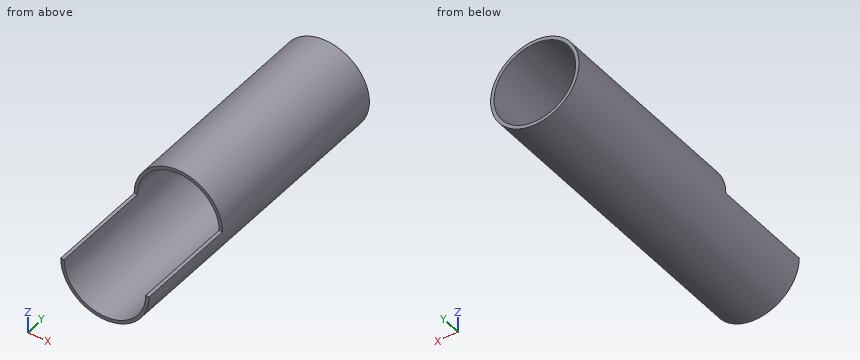
from build123d import *

# Parameters (mm, degrees)
SKETCH1_R           = 25.4
BOSS_EXTRUDE1_DEPTH = 180
SKETCH2_R           = 23.45
CUT_EXTRUDE1_DEPTH  = 180
SKETCH4_W           = 79.8
SKETCH4_H           = 60
CUT_EXTRUDE2_DEPTH  = 50


with BuildPart() as part:
    # Sketch1 → Boss-Extrude1 (new body)
    with BuildSketch(Plane(origin=(0, 0, 0), x_dir=(1, 0, 0), z_dir=(0, 1, 0))):
        with Locations(Location((0, 0, 0), (0, 0, 180))):
            Circle(SKETCH1_R)
    extrude(amount=BOSS_EXTRUDE1_DEPTH)

    # Sketch2 → Cut-Extrude1 (cut)
    with BuildSketch(Plane(origin=(0, 180, 0), x_dir=(1, 0, 0), z_dir=(0, 1, 0))):
        with Locations(Location((0, 0, 0), (0, 0, 270))):
            Circle(SKETCH2_R)
    extrude(amount=-CUT_EXTRUDE1_DEPTH, mode=Mode.SUBTRACT)

    # Sketch4 → Cut-Extrude2 (cut)
    with BuildSketch(Plane.XY.offset(50)):
        with Locations((0, 30)):
            Rectangle(SKETCH4_W, SKETCH4_H)
    extrude(amount=-CUT_EXTRUDE2_DEPTH, mode=Mode.SUBTRACT)


solid = part.part
Here's how the part is built. I have some questions about the finished solid (model axes, mm). Give positions to 0.01 mm unless a question says otherwise; leave off trailing zeros. Loops run counter-clockwise (first coordinate to the right, second up) from the corner with the lowest first, then second, coordinate; pieces in that order, holes last. Notation, with made-up numbers: (48.5, 71) -> (81.5, 71) arc R22 ccw to (81.5, 78) -> close; hole circle Ø6 at (35, -40). An arc over 180 degrees is marked (long way). Answer as a JSON object with one key per item and string values. Group by question number.
Item 1: Imagine slicing it at B-B on z = 8.5. Write out the boundary of the cut face in (x, y).
Item 2: Imagine slicing it at D-D on y = 157. Write out the boundary of the cut face in (x, z).
Item 3: Imagine slicing it at A-A on x = 0. Write out the boundary of the cut face in (y, z), then the cut area to 3 significant figures.
Item 4: Will these pins go through, and if not, where does the flat tip stop? pin 1 (2 mm diameter, centred on y = 134.5, z = -16.5, fed in from -X); pin 2 (3 mm diameter, centred on x = 2, y = 84.5, fed in from -Z); pin 3 (1 mm diameter, centred on x = -24, y = 41.5, fed in from +Z).
Item 5: Imagine slicing it at C-C on y = 45.5. Write out the boundary of the cut face in (x, z).
Item 6: I need wall thicknesses on L1, parallel to X at y = 111, z = 0; L2, parallel to Y at x = 14, z = 19. Which ranges of each line are inside material? Lowest first, please.
Answer list:
{
 "1": {"outline": "(-23.94, 60) -> (-21.86, 60) -> (-21.86, 180) -> (-23.94, 180) -> close; (21.86, 60) -> (23.94, 60) -> (23.94, 180) -> (21.86, 180) -> close"},
 "2": {"outline": "circle Ø50.8 at (0, 0); hole circle Ø46.9 at (0, 0)"},
 "3": {"outline": "(0, -25.4) -> (180, -25.4) -> (180, -23.45) -> (0, -23.45) -> close; (60, 23.45) -> (180, 23.45) -> (180, 25.4) -> (60, 25.4) -> close", "area": "585 mm2"},
 "4": {"pin 1": "stops at x = -20.12", "pin 2": "stops at z = -25.4", "pin 3": "stops at z = 0"},
 "5": {"outline": "(-25.4, 0) arc R25.4 ccw to (25.4, 0) -> (23.45, 0) arc R23.45 cw to (-23.45, 0) -> close"},
 "6": {"L1": "x = -25.4 to -23.45, 23.45 to 25.4", "L2": "y = 60 to 180"}
}
